CAD build for the part. Positions are in the model's coordinates, mm. A direction names the side the tool comes from. Coordinates: 2 decimals unless noted, no trailing zeros. Write each loop counter-clockwise with the first axis right and the second up, starting at its lowest first coordinate (ties: lowest second). Pieces come first, ordered by that corner, then holes.
```python
from build123d import *

# Parameters (mm, degrees)
SKETCH2_W               = 6
SKETCH2_H               = 12
SKETCH2_W_2             = 20
SKETCH2_H_2             = 6
BOSS_EXTRUDE1_DEPTH     = 10
SKETCH6_R               = 1
CUT_EXTRUDE2_DEPTH      = 16.362291496
CUT_EXTRUDE4_DEPTH      = 16.362291496
CUT_EXTRUDE4_DEPTH_BACK = 16.362291496
SKETCH7_R               = 1.625
FILLET1_R               = 1


with BuildPart() as part:
    # Sketch2 → Boss-Extrude1 (new body)
    with BuildSketch(Plane(origin=(0, 0, 0), x_dir=(1, 0, 0), z_dir=(0, 1, 0))):
        Rectangle(SKETCH2_W, SKETCH2_H)
        with Locations((0, -2)):
            Rectangle(SKETCH2_W_2, SKETCH2_H_2)
    extrude(amount=BOSS_EXTRUDE1_DEPTH)

    # Sketch6 → Cut-Extrude2 (cut, through all)
    with BuildSketch(Plane(origin=(0, 0, 0), x_dir=(1, 0, 0), z_dir=(0, 1, 0))):
        with Locations(Location((0, 3, 0), (0, 0, 270))):
            Circle(SKETCH6_R)
        with Locations(Location((0, -2, 0), (0, 0, 270))):
            Circle(SKETCH6_R)
    extrude(amount=CUT_EXTRUDE2_DEPTH, mode=Mode.SUBTRACT)

    # Sketch7 → Cut-Extrude4 (cut, two sides: drawn at the far end of the back side and taken through both)
    with BuildSketch(Plane.XY.offset(-CUT_EXTRUDE4_DEPTH_BACK)):
        with Locations((-7.5, 7.5)):
            Circle(SKETCH7_R)
        with Locations((7.5, 7.5)):
            Circle(SKETCH7_R)
        with BuildLine():
            Line((-10, 0), (-3, 0))
            Line((-3, 0), (-3, 4))
            ThreePointArc((-3, 4), (-3.292893219, 4.707106781), (-4, 5))
            Line((-4, 5), (-10, 5))
            Line((-10, 5), (-10, 0))
        make_face()
        with BuildLine():
            Line((3, 0), (3, 4))
            ThreePointArc((3, 4), (3.292893219, 4.707106781), (4, 5))
            Line((4, 5), (10, 5))
            Line((10, 5), (10, 0))
            Line((10, 0), (3, 0))
        make_face()
    extrude(amount=CUT_EXTRUDE4_DEPTH + CUT_EXTRUDE4_DEPTH_BACK, mode=Mode.SUBTRACT)

    # Fillet1
    fillet1_edges = [part.edges().sort_by_distance(p)[0] for p in [
        (10, 5, 2),
        (10, 10, 2),
        (-10, 5, 2),
        (-10, 10, 2),
        (-3, 7, 5),
        (3, 7, 5),
        (3, 7, -1),
        (-3, 7, -1),
    ]]
    fillet(fillet1_edges, radius=FILLET1_R - 0.0001)  # a hair under: the kernel refuses the full size


solid = part.part
```
Item 1: Two-plate mould, pull along X, no slides. Class faces 1 (the flat face through (-5.7, 7.5, -1)), 2 (the flat face through (-10, 7, 2)), 3 (the cylindrical face through (-7.71, 9.11, 1.96)): +X half, -X half, draft (parallel to the pull), parting line (faces both ways), or undercut.
Item 2: Flat gauge pins, fed straight in: pin 1 Ø1.5 at (x, y) = (5.5, 8) entering from +Z; pin 2 Ø1.9 at (x, y) = (7.5, 7.5) entering from -Z; pin 3 Ø4 at (y, z) = (4, -3) entering from +X; pin 4 Ø1.5 at (x, z) = (5.5, 2) entering from -Y. Where does each tip first touch, or does it go through?
Item 3: Wall check: line 1 along Z through (x, y) = (0, 6.25); line 2 along X through (y, z) = (2.5, 2); line 3 along X through (y, z) = (8, 2). Give the ranges that are in metal, low to high.
Item 4: Which spindle directions (+Z, -Z, +X, -X, +Y, -Y) get a long thin tool onto all of the face, cutting with end or side? Do faces 4 (the flat face through (6, 5, 2)), 5 (the flat face through (-3, 3.8, -1.2)), 6 (the flat face through (-5.7, 7.5, 5)), 7 (the flat face through (5.6, 7.5, -1)). Say none if no direction does.
Item 5: Saw through at D-D, the plane x = 8. Write the cut outline in (y, z).
Item 6: Saw through at A-A, the plane y = 7.5. State how many separate pieces and enclosed holes the cut face has, and give its area (3 significant figures).
Item 7: Saw through at B-B, the plane z = -0.75. Write the cut outline in (x, y) (3 decimals), and give its area (3 significant figures).
Item 8: Saw through at C-C, the plane z = 2. Write the cut outline in (x, y) (3 decimals).
Working result:
1. face 1: draft
1. face 2: -X half
1. face 3: undercut
2. pin 1: stops at z = 5
2. pin 2: passes through
2. pin 3: stops at x = 3.43
2. pin 4: stops at y = 5
3. line 1: z = -6 to -4, -2 to 1, 3 to 6
3. line 2: x = -3 to -1, 1 to 3
3. line 3: x = -10 to -9.05, -5.95 to -1, 1 to 5.95, 9.05 to 10
4. face 4: +Z, -Z, +X, -Y
4. face 5: -Z, -X, -Y
4. face 6: +Z, -X, +Y, -Y
4. face 7: -Z, +X, +Y, -Y
5. outline: (5, -1) - (5.95, -1) - (5.95, 5) - (5, 5) - close; (9.05, -1) - (10, -1) - (10, 5) - (9.05, 5) - close
6. separate pieces: 3
6. enclosed holes: 2
6. area: 112 mm2
7. outline: (-10, 6) arc R1 ccw to (-9, 5) - (-4, 5) arc R1 cw to (-3, 4) - (-3, 0) - (3, 0) - (3, 4) arc R1 cw to (4, 5) - (9, 5) arc R1 ccw to (10, 6) - (10, 9) arc R1 ccw to (9, 10) - (-9, 10) arc R1 ccw to (-10, 9) - close; hole circle Ø3.25 at (-7.5, 7.5); hole circle Ø3.25 at (7.5, 7.5)
7. area: 113 mm2
8. outline: (-10, 6) arc R1 ccw to (-9, 5) - (-4, 5) arc R1 cw to (-3, 4) - (-3, 0) - (-1, 0) - (-1, 10) - (-9, 10) arc R1 ccw to (-10, 9) - close; (1, 0) - (3, 0) - (3, 4) arc R1 cw to (4, 5) - (9, 5) arc R1 ccw to (10, 6) - (10, 9) arc R1 ccw to (9, 10) - (1, 10) - close; hole circle Ø3.25 at (-7.5, 7.5); hole circle Ø3.25 at (7.5, 7.5)
